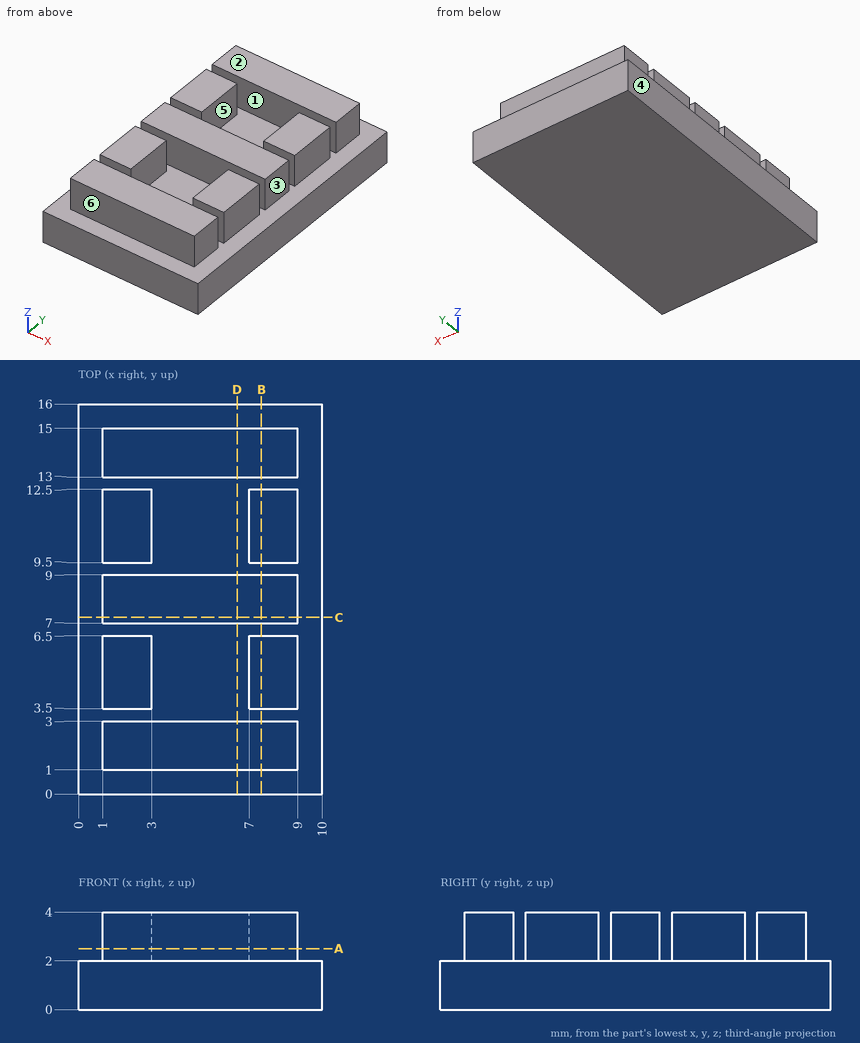
Verification items for this drawing (mm, ordinates from the low corner). A direction names the side the tool comes from. Give positions to 0.01 mm unless a question says otherwise; leave off trailing zeros. Loops run counter-clockwise (first coordinate to the right, second up) from the corner with the lowest first, then second, coordinate; pieces in that order, holes last. Notation, with made-up numbers: (59, 24) - (115, 24) arc R24 cw to (115, 51) - close; hole circle Ø10 at (70, 72). An arc over 180 degrees is marked (long way). Write item = value, one per line. Start each with the question number.
Q1. Cross-section at B-B, the plane x = 7.5. Enter the section's corners in (y, z).
Q2. Thickness scan on line 1 (Y direction, x = 7.5, z = 3.65); line 2 (Y direction, x = 4.5, z = 3.8); line 3 (X direction, y = 12, z = 2.7). Record the ranges inside material, lowest first.
Q3. Cross-section at C-C, the plane y = 7.25. Enter the section's corners in (x, z).
Q4. Tool access check on the marked faces 1, 2 and 3. Record the directions out of +Z, -Z, +X, -X, +Y, -Y that give a thin tool (end or side, any length) a straight path to the whole face; none if there is none.
Q5. Cross-section at D-D, the plane x = 6.5. Enter the section's corners in (y, z), and give its area (3 significant figures).
Q6. Depth check by flat-ended pin: P1, Ø0.6, axis at y = 10.5, z = 3, coming from the -X side; P2, Ø1, axis at x = 3, z = 3.5, coming from the -Y side; P3, Ø0.6, axis at y = 8, z = 3.5, coming from the +X side. Enter the tip coordinate at first touch or a pass-through.
Q7. Cross-section at A-A, the plane z = 2.5. Enter the section's corners in (x, y), and give its area (3 significant figures).
Q8. Mould release check, pull along Y, two halves, no side actions. Record for the marked faces 4, 5 and 6: released by +Y, released by -Y, zero draft, split by the parting line, or undercut.
Answer key:
q1.outline = (0, 0) - (16, 0) - (16, 2) - (15, 2) - (15, 4) - (13, 4) - (13, 2) - (12.5, 2) - (12.5, 4) - (9.5, 4) - (9.5, 2) - (9, 2) - (9, 4) - (7, 4) - (7, 2) - (6.5, 2) - (6.5, 4) - (3.5, 4) - (3.5, 2) - (3, 2) - (3, 4) - (1, 4) - (1, 2) - (0, 2) - close
q2.line_1 = 1 to 3, 3.5 to 6.5, 7 to 9, 9.5 to 12.5, 13 to 15
q2.line_2 = 1 to 3, 7 to 9, 13 to 15
q2.line_3 = 1 to 3, 7 to 9
q3.outline = (0, 0) - (10, 0) - (10, 2) - (9, 2) - (9, 4) - (1, 4) - (1, 2) - (0, 2) - close
q4.face_1 = +Z, +X, -X
q4.face_2 = +Z, +X, -X, +Y, -Y
q4.face_3 = +Z, +X, +Y, -Y
q5.outline = (0, 0) - (16, 0) - (16, 2) - (15, 2) - (15, 4) - (13, 4) - (13, 2) - (9, 2) - (9, 4) - (7, 4) - (7, 2) - (3, 2) - (3, 4) - (1, 4) - (1, 2) - (0, 2) - close
q5.area = 44.0 mm^2
q6.P1 = 1
q6.P2 = 1
q6.P3 = 9
q7.outline = (1, 1) - (9, 1) - (9, 3) - (1, 3) - close; (1, 3.5) - (3, 3.5) - (3, 6.5) - (1, 6.5) - close; (1, 7) - (9, 7) - (9, 9) - (1, 9) - close; (1, 9.5) - (3, 9.5) - (3, 12.5) - (1, 12.5) - close; (1, 13) - (9, 13) - (9, 15) - (1, 15) - close; (7, 3.5) - (9, 3.5) - (9, 6.5) - (7, 6.5) - close; (7, 9.5) - (9, 9.5) - (9, 12.5) - (7, 12.5) - close
q7.area = 72.0 mm^2
q8.face_4 = zero draft
q8.face_5 = undercut
q8.face_6 = released by -Y
